Geometry: final body of the model. Coordinates: model frame, mm. A direction names the side the tool comes from. Round coordinates to 2 decimals unless told otherwise and drop trailing zeros. Loops run counter-clockwise (first coordinate to the right, second up) from the corner with the lowest first, then second, coordinate; pieces in that order, holes last. Notation, with made-up numbers: (62.5, 87) -> (121.5, 87) arc R17 cw to (121.5, 96) -> close; hole circle Ø10 at (80.5, -14.5). An arc over 180 degrees is marked (long way). Answer in a Markdown table with one row per item.
```python
from build123d import *

# Parameters (mm, degrees)
F0_R     = 5
F0_R_2   = 2.45
F1_DEPTH = 4
F3_W     = 1
F3_H     = 1
F5_R     = 0.1
F6_SIZE  = 0.2


with BuildPart() as f1:
    # F0 (on Front) → F1 (new body)
    with BuildSketch(Plane.XZ):
        Circle(F0_R)
        Circle(F0_R_2, mode=Mode.SUBTRACT)
    extrude(amount=F1_DEPTH)

    # F3 (on Top) → F4 (revolve, cut)
    with BuildSketch(Plane.XY):
        with Locations((-3.95, 0.2)):
            Rectangle(F3_W, F3_H)
        with Locations((-3.95, -4.2)):
            Rectangle(F3_W, F3_H)
    revolve(axis=Axis((0, -5.5422200821, 0), (0, -1, 0)), mode=Mode.SUBTRACT)

    # F5
    f5_edges = [f1.edges().sort_by_distance(p)[0] for p in [
        (4.45, 0, 0),
        (3.45, 0, 0),
        (4.45, -4, 0),
        (3.45, -4, 0),
    ]]
    fillet(f5_edges, radius=F5_R)

    # F6
    f6_edges = [f1.edges().sort_by_distance(p)[0] for p in [
        (-5, -4, 0),
        (-5, 0, 0),
    ]]
    chamfer(f6_edges, length=F6_SIZE)


solid = f1.part
```
Item 1: Draft query along X for faces 3 (the face through (-1.08, -1.97, -4.88)), 4 (the face through (-2, -4, -2)), 5 (the face through (-2, -3.7, 3)). Return one class per face: pulls with the +X half, pulls with the -X half, needs draft (parallel to the pull), parting line crosses it, or undercut.
Answer:
| item | result |
|---|---|
| face 3 | parting line crosses it |
| face 4 | needs draft |
| face 5 | undercut |
Item 2: Reachability of faces 1 (the face through (-2, -0.3, 3)), 2 (the face through (-0.5, -2, -2.4)) from +Z, -Z, +X, -X, +Y, -Y: full face, straight path, thin tool, end or side. Return the list, or none.
Answer:
| item | result |
|---|---|
| face 1 | +Y |
| face 2 | +Y, -Y |
Item 3: Line query: probe 1 along Z at (x, y) = (0, -3.65); probe 2 along Y at (x, z) = (-2.25, 3.5); probe 3 along X at (y, z) = (-1.8, -0.75). Output: solid intervals per line, ascending. Write a range as [from, to].
Answer:
| item | result |
|---|---|
| probe 1 | z = [-5, -2.45], [2.45, 5] |
| probe 2 | y = [-3.7, -0.3] |
| probe 3 | x = [-4.94, -2.33], [2.33, 4.94] |
Item 4: Pin query (flat end, axial travel): pin 1 Ø1.5 at (x, z) = (-2.5, 0.5) entering from +Y; pin 2 Ø1.5 at (y, z) = (-3, 2.5) entering from -X; pin 3 Ø1 at (y, z) = (-3, 2.5) entering from +X; pin 4 Ø1.5 at (y, z) = (-1.5, -2) entering from -X. Return the tip coordinate at first contact, or that it passes through.
Answer:
| item | result |
|---|---|
| pin 1 | stops at y = 0 |
| pin 2 | stops at x = -4.68 |
| pin 3 | stops at x = 4.58 |
| pin 4 | stops at x = -4.84 |
Item 5: Cut plane A-A (y = -3.5). Output: boundary loops of the cut face in (x, z), then the cut area to 3 significant figures.
Answer:
| item | result |
|---|---|
| outline | circle Ø10 at (0, 0); hole circle Ø4.9 at (0, 0) |
| area | 59.7 mm² |
